Source: CAD feature listing. Evaluate the final solid. Frame: model axes, mm. Give positions to 0.01 mm unless a question says otherwise; leave off trailing zeros. Loops run counter-clockwise (first coordinate to the right, second up) from the corner with the lowest first, then second, coordinate; pieces in that order, holes last. Notation, with made-up numbers: M -4,9.5 L 28,9.5 A8 cw 28,23.5 Z; hole C 24.5,72.5 d4. An arc over 180 degrees is marked long. Answer in a Markdown table with one row per item.
```python
from build123d import *

# Parameters (mm, degrees)
EXTRUDE_1_DEPTH     = 4
SKETCH_2_R          = 1.5
CUT_EXTRUDE_1_DEPTH = 4
SKETCH_3_R          = 1.5
CUT_EXTRUDE_2_DEPTH = 4
CUT_EXTRUDE_3_DEPTH = 10
CUT_EXTRUDE_5_DEPTH = 10
CUT_EXTRUDE_6_DEPTH = 10
FILLET_1_R          = 3


with BuildPart() as part:
    # 草图1 → 凸台-拉伸1 (new body)
    with BuildSketch(Plane(origin=(0, 0, 0), x_dir=(1, 0, 0), z_dir=(0, 1, 0))):
        Polygon((100, 150), (75, 0), (0, 0), (0, 150), align=None)
    extrude(amount=EXTRUDE_1_DEPTH)

    # 草图2 → 切除-拉伸1 (cut)
    with BuildSketch(Plane(origin=(0, 4, 0), x_dir=(1, 0, 0), z_dir=(0, 1, 0))):
        with Locations(Location((10, 25, 0), (0, 0, 270))):
            Circle(SKETCH_2_R)
        with Locations(Location((34, 55, 0), (0, 0, 270))):
            Circle(SKETCH_2_R)
        with Locations(Location((34, 25, 0), (0, 0, 270))):
            Circle(SKETCH_2_R)
        with Locations(Location((10, 55, 0), (0, 0, 270))):
            Circle(SKETCH_2_R)
    extrude(amount=-CUT_EXTRUDE_1_DEPTH, mode=Mode.SUBTRACT)

    # 草图3 → 切除-拉伸2 (cut)
    with BuildSketch(Plane(origin=(0, 4, 0), x_dir=(1, 0, 0), z_dir=(0, 1, 0))):
        with Locations(Location((10, 142.5, 0), (0, 0, 270))):
            Circle(SKETCH_3_R)
        with Locations(Location((36, 142.5, 0), (0, 0, 270))):
            Circle(SKETCH_3_R)
        with Locations(Location((57, 142.5, 0), (0, 0, 270))):
            Circle(SKETCH_3_R)
        with Locations(Location((83, 142.5, 0), (0, 0, 270))):
            Circle(SKETCH_3_R)
    extrude(amount=-CUT_EXTRUDE_2_DEPTH, mode=Mode.SUBTRACT)

    # 草图4 → 切除-拉伸3 (cut)
    with BuildSketch(Plane(origin=(0, 4, 0), x_dir=(1, 0, 0), z_dir=(0, 1, 0))):
        Polygon((121.630506201, 0), (50, 0), (50, 90), (150.537772798, 90), align=None)
    extrude(amount=-CUT_EXTRUDE_3_DEPTH, mode=Mode.SUBTRACT)

    # 草图5 → 切除-拉伸5 (cut)
    with BuildSketch(Plane(origin=(0, 4, 0), x_dir=(1, 0, 0), z_dir=(0, 1, 0))):
        Polygon((150.2124031, 125.352298199), (66.770540327, 64.546264366), (50, 90), (96.666666667, 130), align=None)
    extrude(amount=-CUT_EXTRUDE_5_DEPTH, mode=Mode.SUBTRACT)

    # 草图6 → 切除-拉伸6 (cut)
    with BuildSketch(Plane(origin=(0, 4, 0), x_dir=(1, 0, 0), z_dir=(0, 1, 0))):
        Polygon((96.666666667, 130), (140.554271479, 130), (107.506476867, 160.861157787), (96.666666667, 160.861157787), align=None)
    extrude(amount=-CUT_EXTRUDE_6_DEPTH, mode=Mode.SUBTRACT)

    # 圆角1
    fillet_1_edges = [part.edges().sort_by_distance(p)[0] for p in [
        (50, 2, -90),
        (50, 2, 0),
        (96.666666667, 2, -130),
        (0, 2, -150),
        (0, 2, 0),
        (96.666666667, 2, -150),
    ]]
    fillet(fillet_1_edges, radius=FILLET_1_R)


solid = part.part
```
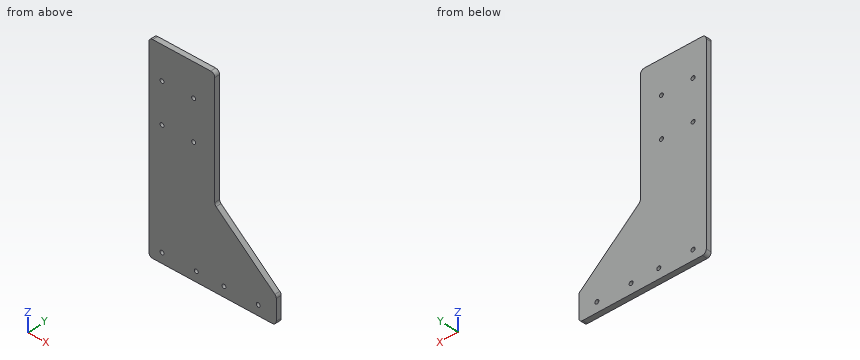
1) Section C-C, the plane x = 57. Return loops of the section in (y, z).
Reply:
| item | result |
|---|---|
| outline | M 0,-150 L 4,-150 L 4,-144 L 0,-144 Z; M 0,-141 L 4,-141 L 4,-96 L 0,-96 Z |
2) Section D-D, the plane z = -25. Return loops of the section in (x, y), then the cut area to 3 significant figures.
Reply:
| item | result |
|---|---|
| outline | M 0,0 L 8.5,0 L 8.5,4 L 0,4 Z; M 11.5,0 L 32.5,0 L 32.5,4 L 11.5,4 Z; M 35.5,0 L 50,0 L 50,4 L 35.5,4 Z |
| area | 176 mm² |
3) Section B-B, the plane y = 3.2. Count the separate pieces of the cut face and the enclosed holes in it, then the cut area to 3 significant figures.
Reply:
| item | result |
|---|---|
| separate pieces | 1 |
| enclosed holes | 8 |
| area | 9,300 mm² |
4) Material intervals for L1, parallel to X at y = 2.2, z = -25; L2, parallel to X at y = 0.9, z = -142.5; L3, parallel to X at y = 2.2, z = -25.5, sorted ascending.
Reply:
| item | result |
|---|---|
| L1 | x = 0 to 8.5, 11.5 to 32.5, 35.5 to 50 |
| L2 | x = 0 to 8.5, 11.5 to 34.5, 37.5 to 55.5, 58.5 to 81.5, 84.5 to 96.67 |
| L3 | x = 0 to 8.59, 11.41 to 32.59, 35.41 to 50 |
5) Pin query (flat end, axial travel): pin 1 Ø1 at (y, z) = (2.5, -53.5) entering from +X. Return the tip coordinate at first contact, or that it passes through.
Reply:
| item | result |
|---|---|
| pin 1 | stops at x = 50 |
6) Section A-A, the plane x = 10. Return loops of the section in (y, z), then the cut area to 3 significant figures.
Reply:
| item | result |
|---|---|
| outline | M 0,-150 L 4,-150 L 4,-144 L 0,-144 Z; M 0,-141 L 4,-141 L 4,-56.5 L 0,-56.5 Z; M 0,-53.5 L 4,-53.5 L 4,-26.5 L 0,-26.5 Z; M 0,-23.5 L 4,-23.5 L 4,0 L 0,0 Z |
| area | 564 mm² |
